Part model, mm, in its own coordinate system. Face numbers are marked on the shaded views. A direction names the side the tool comes from. Round coordinates to 2 decimals unless told otherwise and drop trailing zeros. Order: outer loops, then holes, each group sorted by start corner. A loop starts at its lowest first (then second) coordinate and runs counter-clockwise, first axis right, second up. Notation, with made-up numbers: (58.5, 16) -> (73.5, 16) arc R16 ccw to (73.5, 20) -> close; hole circle Ø3 at (39.25, 82.25). An arc over 180 degrees is marked (long way). Answer as a JSON object with one key per item and string values. Group by question number.
Autodesk Inventor part; units mm, degrees
ref_plane "YZ Plane" through (0, 0, 0) normal (1, 0, 0) x (0, 1, 0)
ref_plane "XZ Plane" through (0, 0, 0) normal (0, 1, 0) x (-1, 0, 0)
ref_plane "XY Plane" through (0, 0, 0) normal (0, 0, 1) x (1, 0, 0)
sketch "Sketch1" plane through (0, 0, 0) normal (0, 1, 0) x (-1, 0, 0)
  line L0 (0, 0) -> (9.525, 0)
  line L1 (9.525, 0) -> (9.525, -114.3)
  line L2 (9.525, -114.3) -> (0, -114.3)
  line L3 (0, -114.3) -> (0, 0)
  dimension "d0" = 9.525
  dimension "d1" = 114.3
extrude "Extrusion1" add sketch "Sketch1" along normal blind 9.525
sketch "Sketch2" plane through (0, 9.525, 0) normal (0, 1, 0) x (1, 0, 0)
  point P0 (0, 0)
sketch "Sketch3" plane through (0, 0, 0) normal (1, 0, 0) x (0, 0, -1)
  circle A0 centre (4.7752, 4.7625) radius 3.175
  circle A1 centre (109.7788, 4.7625) radius 3.175
  point P0 (0, 0)
  dimension "d4" = 6.35
  dimension "d5" = 6.35
hole "Hole1" at (0, 4.7625, -109.7788) at (0, 4.7625, -4.7752) direction (-1, 0, 0) diameter 6.35 depth 6.35
sketch "Sketch4" plane through (0, 9.525, 0) normal (0, 1, 0) x (1, 0, 0)
  line L0 (-6.35, 106.6038) -> (0, 106.6038)
  line L1 (-6.35, 1.6002) -> (-6.35, 7.9502)
  line L2 (-3.175, 106.6038) -> (-6.35, 106.6038)
  line L3 (-6.35, 106.6038) -> (-6.35, 7.9502)
  line L4 (-6.35, 7.9502) -> (-3.175, 7.9502)
  line L5 (-3.175, 7.9502) -> (-3.175, 106.6038)
  point P0 (0, 0)
extrude "Extrusion2" cut sketch "Sketch4" against normal blind 12.7
sketch "Sketch5" plane through (0, 9.525, 0) normal (0, 1, 0) x (1, 0, 0)
  line L0 (-6.35, 106.6038) -> (-6.35, 7.9502)
  line L1 (-3.175, 7.9502) -> (-6.35, 7.9502)
  line L2 (-6.35, 7.9502) -> (-6.35, 11.1252)
  line L3 (-6.35, 11.1252) -> (-3.175, 11.1252)
  line L4 (-3.175, 11.1252) -> (-3.175, 7.9502)
  line L5 (-6.35, 106.6038) -> (-3.175, 106.6038)
  line L6 (-3.175, 106.6038) -> (-6.35, 106.6038)
  line L7 (-6.35, 106.6038) -> (-6.35, 103.4499)
  line L8 (-6.35, 103.4499) -> (-3.175, 103.4499)
  line L9 (-3.175, 103.4499) -> (-3.175, 106.6038)
  point P0 (0, 0)
  dimension "d15" = 3.175
extrude "Extrusion3" add sketch "Sketch5" against normal blind 9.525
sketch "Sketch6" plane through (-9.525, 0, -114.3) normal (-1, 0, 0) x (0, 0, 1)
  point P0 (114.3, 0)
sketch "Sketch7" plane through (-9.525, 0, -114.3) normal (-1, 0, 0) x (0, 0, 1)
  line L0 (10.8501, 9.525) -> (10.8501, 0)
  line L1 (10.8501, 6.3627) -> (20.6362, 6.3627)
  line L2 (20.6362, 3.1877) -> (10.8501, 3.1877)
  line L3 (10.8501, 3.1877) -> (10.8501, 6.3627)
  line L4 (103.1748, 9.525) -> (103.1748, 0)
  line L5 (10.8501, 6.3627) -> (103.1748, 6.3627)
  line L6 (103.1748, 6.3627) -> (103.1748, 3.1877)
  line L7 (103.1748, 3.1877) -> (10.8501, 3.1877)
  line L8 (10.8501, 3.1877) -> (10.8501, 6.3627)
  point P0 (114.3, 0)
  point P1 (10.8501, 4.7625)
  dimension "d18" = 3.175
sketch "Sketch8" plane through (-9.525, 0, -114.3) normal (-1, 0, 0) x (0, 0, 1)
  point P0 (114.3, 0)
ref_plane "Work Plane1" through (-9.525, 3.1877, -11.1252) normal (0, 1, 0) x (0, 0, -1)
sketch "Sketch9" plane through (-9.525, 3.1877, -11.1252) normal (0, 1, 0) x (0, 0, -1)
  point P0 (-11.1252, -9.525)
sketch "Sketch10" plane through (-9.525, 3.1877, -11.1252) normal (0, 1, 0) x (0, 0, -1)
  line L0 (-11.1252, 0) -> (103.1748, 0)
  arc A0 (92.2109, 0) -> (0.0002, 0) centre (46.1056, 0.3232) ccw
  line L1 (92.2109, 0) -> (0.0002, 0)
  line L2 (92.3247, -3.175) -> (0, -3.175)
  point P0 (-11.1252, -9.525)
  point P1 (-11.1252, -9.525)
  point P2 (-11.1252, -9.525)
extrude "Extrusion4" add sketch "Sketch10" along normal blind 3.175
sketch "Sketch11" plane through (-9.525, 3.1877, -11.1252) normal (0, -1, 0) x (1, 0, 0)
  arc A0 (0, -0.0002) -> (0, -92.2109) centre (-0.3232, -46.1056) ccw
  line L0 (-46.4297, -46.1056) -> (-33.7222, -46.1056)
  point P0 (9.525, 11.1252)
sketch "Sketch12" plane through (-9.525, 3.1877, -11.1252) normal (0, -1, 0) x (1, 0, 0)
  point P0 (9.525, 11.1252)
sketch "Sketch13" plane through (-9.525, 3.1877, -11.1252) normal (0, -1, 0) x (1, 0, 0)
  circle A0 centre (-33.7224, -46.1055) radius 3.175
  point P0 (9.525, 11.1252)
  dimension "d22" = 6.35
extrude "Extrusion5" cut sketch "Sketch13" against normal blind 3.175
properties part number "MTV Truning Connecter (10.7)"
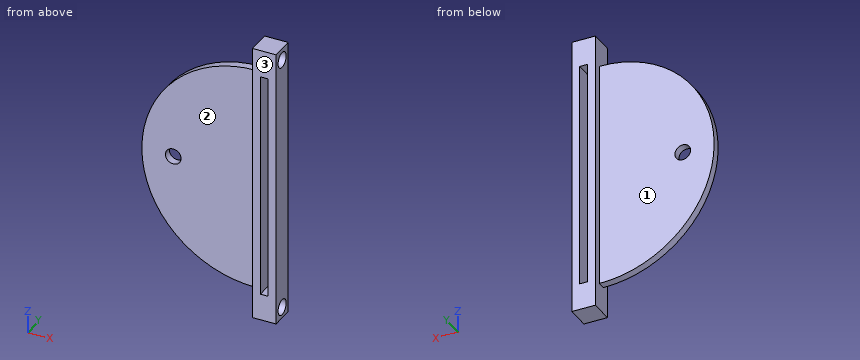
Q1. Drop flat-ended pins along their axis: pin 1 Ø3 at (x, z) = (-30.5, -33.5) entering from +Y; pin 2 Ø5 at (y, z) = (4.76, -109.78) entering from +X; pin 3 Ø8 at (x, z) = (-39, -85.5) entering from -Y. Give the stop position or say it passes through.
Q2. Band-saw the part on A-A (z = -19). List the corners of the cut face in (x, y) (3 decimals).
Q3. Wall check: line 1 (X direction, y = 2, z = -61) (3 decimals); line 2 (Z direction, x = -3, y = 2.75); line 3 (Y direction, x = -18, z = -99.5). Give the ranges that are in metal, low to high. Write a range as [from, to].
Q4. Band-saw the part on C-C (z = -35). List the corners of the cut face in (x, y) (3 decimals), plus the area to 3 significant figures.
Q5. Which spindle directions (+Z, -Z, +X, -X, +Y, -Y) get a long thin tool onto all of the face, cutting with end or side? Do the marked faces 1, 2 and 3. Say none if no direction does.
Q6. Band-saw the part on D-D (x = -24). List the corners of the cut face in (y, z), plus the area to 3 significant figures.
Q7. Band-saw the part on B-B (x = -44). List the corners of the cut face in (y, z).
Completed:
{
 "1": {"pin 1": "y = 6.36", "pin 2": "x = -6.35", "pin 3": "y = 3.19"},
 "2": {"outline": "(-35.621, 3.188) -> (-9.525, 3.188) -> (-9.525, 0) -> (-6.35, 0) -> (-6.35, 9.525) -> (-9.525, 9.525) -> (-9.525, 6.363) -> (-35.621, 6.363) -> close; (-3.175, 0) -> (0, 0) -> (0, 9.525) -> (-3.175, 9.525) -> close"},
 "3": {"line 1": "[-9.525, -6.35], [-3.175, 0]", "line 2": "[-114.3, -112.23], [-107.32, -7.23], [-2.32, 0]", "line 3": "[3.19, 6.36]"},
 "4": {"outline": "(-50.241, 3.188) -> (-9.525, 3.188) -> (-9.525, 0) -> (-6.35, 0) -> (-6.35, 9.525) -> (-9.525, 9.525) -> (-9.525, 6.363) -> (-50.241, 6.363) -> close; (-3.175, 0) -> (0, 0) -> (0, 9.525) -> (-3.175, 9.525) -> close", "area": "190 mm2"},
 "5": {"face 1": "+Z, -Z, -X, +Y", "face 2": "+Z, -Z, -X, -Y", "face 3": "+Z, -Z, +X, -X, -Y"},
 "6": {"outline": "(3.19, -101.11) -> (6.36, -101.11) -> (6.36, -13.35) -> (3.19, -13.35) -> close", "area": "279 mm2"},
 "7": {"outline": "(3.19, -88.21) -> (6.36, -88.21) -> (6.36, -60.32) -> (3.19, -60.32) -> close; (3.19, -54.15) -> (6.36, -54.15) -> (6.36, -26.26) -> (3.19, -26.26) -> close"}
}
